Design review of the part built by this model. Coordinates are the model's own, in mm. A direction names the side the tool comes from. Round coordinates to 2 decimals unless told otherwise and drop trailing zeros. Order: outer loops, then holes, each group sorted by start corner. A loop starts at its lowest first (then second) coordinate and runs counter-clockwise, first axis right, second up. Notation, with made-up numbers: (39, -2.5) - (51, -2.5) arc R28 cw to (51, 34.5) - close; hole circle Ø1 at (49, 53.25). An arc over 180 degrees is marked (long way). Use CSV: the item, a comma, the result in double quotes. Start each with the question number.
from build123d import *


with BuildPart() as part:
    # Esquisse1 → R_volution1 (revolve)
    with BuildSketch(Plane.XY, mode=Mode.PRIVATE) as r_volution1_sk:
        with BuildLine():
            Line((31.5, 0), (38, 0))
            Line((38, 0), (38, 5.156854249))
            Line((38, 5.156854249), (32, 5.156854249))
            Line((32, 5.156854249), (17.99973552, 19.157118729))
            ThreePointArc((17.99973552, 19.157118729), (16.626709378, 23.64451305), (19.57751766, 27.293436049))
            ThreePointArc((19.57751766, 27.293436049), (21.815123989, 28.31126724), (24, 29.43784579))
            Line((24, 29.43784579), (24, 30))
            Line((24, 30), (3.5, 30))
            Line((3.5, 30), (3.5, 29.242640687))
            ThreePointArc((3.5, 29.242640687), (3.728361402, 28.09459039), (4.378679656, 27.121320344))
            Line((4.378679656, 27.121320344), (31.5, 0))
        make_face()
    revolve(r_volution1_sk.sketch.rotate(Axis((0, 49.284488144, 0), (0, -1, 0)), 90), axis=Axis((0, 49.284488144, 0), (0, -1, 0)))


solid = part.part
Q1. Take a section at A-A (z = 0). State the section outline as (x, y) points.
Q2. Tool access review of faces 1 (the flat face through (-28.3, 0, 14.3)), 2 (the cylindrical face through (-7.21, 29.72, 22.89)): name each direction out of +Z, -Z, +X, -X, +Y, -Y from which nothing blocks a thin tool from reaching the whole face with its end or side.
Q3. Clearance check with flat-ended pins moving along their axes: pin 1 (1 mm diameter, centred on y = 3.5, z = -8, fed in from -X); pin 2 (6 mm diameter, centred on y = 24.5, z = -1.5, fed in from -X); pin 3 (2 mm diameter, centred on x = -0.5, y = 16.5, fed in from +Z); pin 4 (4 mm diameter, centred on x = 0, z = 0, fed in from +Y). State where each tip first meets the part, or that it passes through.
Q4. The part is to be moulded in two halves that separate along X. For faces 3 (the conical face through (11.37, 18.48, -14.82)), 4 (the flat face through (0, 30, 5)), 5 (the conical face through (-2.73, 22.41, 8.67)), 6 (the cylindrical face through (3.105, 29.616, 1.615)), say which applies: +X half, -X half, draft (parallel to the pull), parting line (faces both ways), or undercut.
Q5. Take a section at C-C (y = 13.5). State the section outline as (x, z) points.
Q6. Take a section at B-B (x = 0). State the section outline as (y, z) points.
Q7. Take a section at D-D (y = 2). State the section outline as (x, z) points, plus the area to 3 significant figures.
Q8. For L1, parallel to X at y = 29.6, z = 0; L2, parallel to X at y = 4, z = -3.5; L3, parallel to Y at x = 14.5, z = 14, list the stretches that pass through material, from the lowest coordinate up. Write a range as [from, to].
Findings below:
1,outline,"(-38, 0) - (-31.5, 0) - (-4.38, 27.12) arc R3 ccw to (-3.5, 29.24) - (-3.5, 30) - (-24, 30) - (-24, 29.44) arc R50 ccw to (-19.58, 27.29) arc R5 cw to (-18, 19.16) - (-32, 5.16) - (-38, 5.16) - close; (3.5, 29.24) arc R3 ccw to (4.38, 27.12) - (31.5, 0) - (38, 0) - (38, 5.16) - (32, 5.16) - (18, 19.16) arc R5 cw to (19.58, 27.29) arc R50 ccw to (24, 29.44) - (24, 30) - (3.5, 30) - close"
2,face 1,"+Z, -Z, +X, -X, -Y"
2,face 2,"+Y"
3,pin 1,"stops at x = -37.25"
3,pin 2,"stops at x = -20"
3,pin 3,"stops at z = 21.65"
3,pin 4,"passes through"
4,face 3,"parting line"
4,face 4,"draft"
4,face 5,"undercut"
4,face 6,"undercut"
5,outline,"circle Ø47.31 at (0, 0); hole circle Ø36 at (0, 0)"
6,outline,"(0, -38) - (5.16, -38) - (5.16, -32) - (19.16, -18) arc R5 cw to (27.29, -19.58) arc R50 ccw to (29.44, -24) - (30, -24) - (30, -3.5) - (29.24, -3.5) arc R3 ccw to (27.12, -4.38) - (0, -31.5) - close; (0, 31.5) - (27.12, 4.38) arc R3 ccw to (29.24, 3.5) - (30, 3.5) - (30, 24) - (29.44, 24) arc R50 ccw to (27.29, 19.58) arc R5 cw to (19.16, 18) - (5.16, 32) - (5.16, 38) - (0, 38) - close"
7,outline,"circle Ø76 at (0, 0); hole circle Ø59 at (0, 0)"
7,area,"1,800 mm^2"
8,L1,"x = [-24, -3.5], [3.5, 24]"
8,L2,"x = [-37.84, -27.28], [27.28, 37.84]"
8,L3,"y = [11.34, 17], [27.54, 30]"
